Drawing for the job (mm, zero at the part's lowest x, y, z). A direction names the side the tool comes from. Give positions to 0.01 mm unless a question says otherwise; leave off trailing zeros. Write each loop counter-clockwise with the first axis right and the second up, starting at its lowest first coordinate (ties: lowest second). Pieces come first, ordered by that corner, then holes.
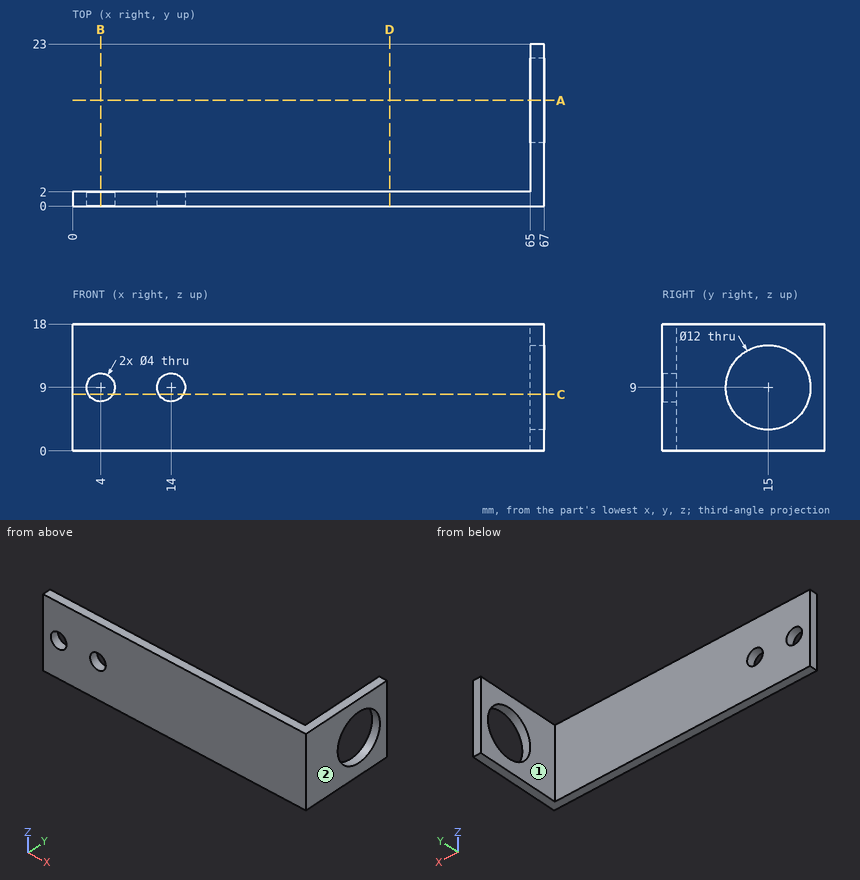
1. Slice it at B-B, the plane x = 4. Write the cut outline in (y, z), and give its area (3 significant figures).
Calculated:
outline: (0, 0) - (2, 0) - (2, 7) - (0, 7) - close; (0, 11) - (2, 11) - (2, 18) - (0, 18) - close
area: 28.0 mm2
2. Slice it at A-A, the plane y = 15. Write the cut outline in (x, z), and give its area (3 significant figures).
Calculated:
outline: (65, 0) - (67, 0) - (67, 3) - (65, 3) - close; (65, 15) - (67, 15) - (67, 18) - (65, 18) - close
area: 12.0 mm2
3. Probe probe 1 along Z at (x, y) = (4, 0.7); probe 2 along Y at (x, z) = (65.6, 9); probe 3 along Y at (x, z) = (53, 3.5). List the from-to ranges inside material, lowest first.
Calculated:
probe 1: z = 0 to 7, 11 to 18
probe 2: y = 0 to 9, 21 to 23
probe 3: y = 0 to 2
4. Pin check, flat tips, straight feed: P1, Ø4, axis at y = 9, z = 8.5, coming from the -X side; P2, Ø3, axis at x = 13, z = 7, coming from the +Y side. Stop position of each tip, or through.
Calculated:
P1: stops at x = 65
P2: stops at y = 2
5. Slice it at D-D, the plane x = 45. Write the cut outline in (y, z), and give its area (3 significant figures).
Calculated:
outline: (0, 0) - (2, 0) - (2, 18) - (0, 18) - close
area: 36.0 mm2
6. Slice it at C-C, the plane z = 8. Write the cut outline in (x, y).
Calculated:
outline: (0, 0) - (2.27, 0) - (2.27, 2) - (0, 2) - close; (5.73, 0) - (12.27, 0) - (12.27, 2) - (5.73, 2) - close; (15.73, 0) - (67, 0) - (67, 9.08) - (65, 9.08) - (65, 2) - (15.73, 2) - close; (65, 20.92) - (67, 20.92) - (67, 23) - (65, 23) - close
7. Which spindle directions (+Z, -Z, +X, -X, +Y, -Y) get a long thin tool onto all of the face, cutting with end or side? Do the marked faces 1 and 2. Say none if no direction does.
Calculated:
face 1: +Z, -Z, -X, +Y
face 2: +Z, -Z, +X, +Y, -Y
